```python
from build123d import *

# Parameters (mm, degrees)
F1_DEPTH  = 30
F0_W      = 37.5
F0_H      = 10
F2_DEPTH  = 100
F4_DEPTH  = 70
F5_W      = 20.9091625453
F5_H      = 25
F6_DEPTH  = 70
F7_DEPTH  = 70
F9_DEPTH  = 5
F12_DEPTH = 17.5


with BuildPart() as f1:
    # F0 (on Right) → F1 (new body)
    with BuildSketch(Plane.YZ):
        with BuildLine():
            Line((-100, 15), (-100, 0))
            Line((-100, 0), (-50, 0))
            Line((-50, 0), (-12.5, 0))
            Line((-12.5, 0), (12.5, 0))
            Line((12.5, 0), (50, 0))
            Line((50, 0), (100, 0))
            Line((100, 0), (100, 40))
            Line((100, 40), (40, 40))
            ThreePointArc((40, 40), (20.4711584909, 13.3855671691), (-12.5, 15))
            Line((-12.5, 15), (-100, 15))
        make_face()
    extrude(amount=-F1_DEPTH)

    # F0 (on Right) → F2 (join)
    with BuildSketch(Plane.YZ):
        with Locations((-31.25, -5)):
            Rectangle(F0_W, F0_H)
        with Locations((31.25, -5)):
            Rectangle(F0_W, F0_H)
    extrude(amount=-F2_DEPTH)

    # F3 (on face) → F4 (join)
    with BuildSketch(Plane(origin=(-30, 0, 0), x_dir=(0, -1, 0), z_dir=(-1, 0, 0))):
        with BuildLine():
            Line((12.5, 15), (-23.473678133, 15))
            ThreePointArc((-23.473678133, 15), (-34.5610974405, 25.633015883), (-40, 40))
            Line((-40, 40), (-100, 40))
            Line((-100, 40), (-100, 0))
            Line((-100, 0), (-50, 0))
            Line((-50, 0), (-12.5, 0))
            Line((-12.5, 0), (12.5, 0))
            Line((12.5, 0), (50, 0))
            Line((50, 0), (100, 0))
            Line((100, 0), (100, 15))
            Line((100, 15), (12.5, 15))
        make_face()
    extrude(amount=F4_DEPTH)

    # F5 (on face) → F6 (join)
    with BuildSketch(Plane(origin=(-100, 0, 0), x_dir=(0, -1, 0), z_dir=(-1, 0, 0))):
        with BuildLine():
            Line((-23.473678133, 15), (-5.478678133, 15))
            Line((-5.478678133, 15), (-38.6573392432, 34.1557089233))
            ThreePointArc((-38.6573392432, 34.1557089233), (-32.7999061901, 23.2030943833), (-23.473678133, 15))
        make_face()
        with Locations((-89.5454187273, 27.5)):
            Rectangle(F5_W, F5_H)
        Polygon((-79.0908374547, 40), (-48.7799483222, 40), (-79.0908374547, 57.5), align=None)
    extrude(amount=-F6_DEPTH)

    # F5 (on face) → F7 (cut)
    with BuildSketch(Plane(origin=(-100, 0, 0), x_dir=(0, -1, 0), z_dir=(-1, 0, 0))):
        with BuildLine():
            Line((-48.7799483222, 40), (-38.6573392432, 34.1557089233))
            ThreePointArc((-38.6573392432, 34.1557089233), (-39.4545948044, 37.048924554), (-40, 40))
            Line((-40, 40), (-48.7799483222, 40))
        make_face()
    extrude(amount=-F7_DEPTH, mode=Mode.SUBTRACT)

    # F8 (on face) → F9 (cut)
    with BuildSketch(Plane(origin=(0, -5.1255209951, 8.8776627788), x_dir=(1, 0, 0), z_dir=(0, -0.5, 0.8660254038))):
        with BuildLine():
            Line((-85.9351158142, 57.2446744423), (-76.4564392374, 57.2446744423))
            ThreePointArc((-76.4564392374, 57.2446744423), (-77.5, 62.2446744423), (-76.4564392374, 67.2446744423))
            Line((-76.4564392374, 67.2446744423), (-85.9351158142, 67.2446744423))
            Line((-85.9351158142, 67.2446744423), (-99.6410161514, 67.2446744423))
            ThreePointArc((-99.6410161514, 67.2446744423), (-99.9101386799, 64.7511096302), (-100, 62.2446744423))
            ThreePointArc((-100, 62.2446744423), (-99.9101386799, 59.7382392545), (-99.6410161514, 57.2446744423))
            Line((-99.6410161514, 57.2446744423), (-85.9351158142, 57.2446744423))
        make_face()
        with BuildLine():
            Line((-60, 73.7011136797), (-60, 96.8856905937))
            ThreePointArc((-60, 96.8856905937), (-62.4935647997, 97.1548131213), (-64.999999975, 97.2446744423))
            ThreePointArc((-64.999999975, 97.2446744423), (-67.5064351754, 97.1548131231), (-70, 96.8856905937))
            Line((-70, 96.8856905937), (-70, 73.7011136797))
            ThreePointArc((-70, 73.7011136797), (-65, 74.7446744423), (-60, 73.7011136797))
        make_face()
        with BuildLine():
            Line((-70, 12.2446744423), (-60, 12.2446744423))
            Line((-60, 12.2446744423), (-60, 50.7882352049))
            ThreePointArc((-60, 50.7882352049), (-65, 49.7446744423), (-70, 50.7882352049))
            Line((-70, 50.7882352049), (-70, 12.2446744423))
        make_face()
        with BuildLine():
            ThreePointArc((-30.3589838486, 57.2446744423), (-30.0898613201, 59.7382392545), (-30, 62.2446744423))
            ThreePointArc((-30, 62.2446744423), (-30.0898613201, 64.7511096302), (-30.3589838486, 67.2446744423))
            Line((-30.3589838486, 67.2446744423), (-53.5435607626, 67.2446744423))
            ThreePointArc((-53.5435607626, 67.2446744423), (-52.7636710884, 64.7985449884), (-52.5, 62.2446744423))
            ThreePointArc((-52.5, 62.2446744423), (-52.7636710884, 59.6908038962), (-53.5435607626, 57.2446744423))
            Line((-53.5435607626, 57.2446744423), (-30.3589838486, 57.2446744423))
        make_face()
        with BuildLine():
            ThreePointArc((-64.999999975, 97.2446744423), (-62.4935647997, 97.1548131213), (-60, 96.8856905937))
            Line((-60, 96.8856905937), (-60, 97.2446744423))
            Line((-60, 97.2446744423), (-64.999999975, 97.2446744423))
        make_face()
        with BuildLine():
            ThreePointArc((-70, 96.8856905937), (-67.5064351754, 97.1548131231), (-64.999999975, 97.2446744423))
            Line((-64.999999975, 97.2446744423), (-70, 97.2446744423))
            Line((-70, 97.2446744423), (-70, 96.8856905937))
        make_face()
        with BuildLine():
            Line((-100, 67.2446744423), (-100, 62.2446744423))
            ThreePointArc((-100, 62.2446744423), (-99.9101386799, 64.7511096302), (-99.6410161514, 67.2446744423))
            Line((-99.6410161514, 67.2446744423), (-100, 67.2446744423))
        make_face()
        with BuildLine():
            Line((-100, 62.2446744423), (-100, 57.2446744423))
            Line((-100, 57.2446744423), (-99.6410161514, 57.2446744423))
            ThreePointArc((-99.6410161514, 57.2446744423), (-99.9101386799, 59.7382392545), (-100, 62.2446744423))
        make_face()
        with BuildLine():
            ThreePointArc((-30.3589838486, 67.2446744423), (-30.0898613201, 64.7511096302), (-30, 62.2446744423))
            Line((-30, 62.2446744423), (-30, 67.2446744423))
            Line((-30, 67.2446744423), (-30.3589838486, 67.2446744423))
        make_face()
        with BuildLine():
            Line((-30.3589838486, 57.2446744423), (-30, 57.2446744423))
            Line((-30, 57.2446744423), (-30, 62.2446744423))
            ThreePointArc((-30, 62.2446744423), (-30.0898613201, 59.7382392545), (-30.3589838486, 57.2446744423))
        make_face()
        with BuildLine():
            ThreePointArc((-70, 50.7882352049), (-65, 49.7446744423), (-60, 50.7882352049))
            ThreePointArc((-60, 50.7882352049), (-56.1611652352, 53.4058396775), (-53.5435607626, 57.2446744423))
            ThreePointArc((-53.5435607626, 57.2446744423), (-52.7636710884, 59.6908038962), (-52.5, 62.2446744423))
            ThreePointArc((-52.5, 62.2446744423), (-52.7636710884, 64.7985449884), (-53.5435607626, 67.2446744423))
            ThreePointArc((-53.5435607626, 67.2446744423), (-56.1611652352, 71.0835092071), (-60, 73.7011136797))
            ThreePointArc((-60, 73.7011136797), (-65, 74.7446744423), (-70, 73.7011136797))
            ThreePointArc((-70, 73.7011136797), (-73.8388347648, 71.0835092071), (-76.4564392374, 67.2446744423))
            ThreePointArc((-76.4564392374, 67.2446744423), (-77.5, 62.2446744423), (-76.4564392374, 57.2446744423))
            ThreePointArc((-76.4564392374, 57.2446744423), (-73.8388347648, 53.4058396775), (-70, 50.7882352049))
        make_face()
    extrude(amount=-F9_DEPTH, mode=Mode.SUBTRACT)

    # F11 (on offset) → F12 (cut)
    with BuildSketch(Plane.XY.offset(57.5)):
        with BuildLine():
            add(Edge.make_bspline(
                [(-65, 79.0908374547), (-100, 79.0908374547), (-100, 48.7799483222)],
                knots=[4.7123889804, 4.7123889804, 4.7123889804, 6.2831853072, 6.2831853072, 6.2831853072], degree=2, weights=[1, 0.7071067812, 1]))
            Line((-65, 79.0908374547), (-100, 79.0908374547))
            Line((-100, 79.0908374547), (-100, 48.7799483222))
        make_face()
        with BuildLine():
            Line((-30, 48.7799483222), (-30, 79.0908374547))
            Line((-30, 79.0908374547), (-65, 79.0908374547))
            add(Edge.make_bspline(
                [(-30, 48.7799483222), (-30, 79.0908374547), (-65, 79.0908374547)],
                knots=[3.1415926536, 3.1415926536, 3.1415926536, 4.7123889804, 4.7123889804, 4.7123889804], degree=2, weights=[1, 0.7071067812, 1]))
        make_face()
    extrude(amount=-F12_DEPTH, mode=Mode.SUBTRACT)


solid = f1.part
```
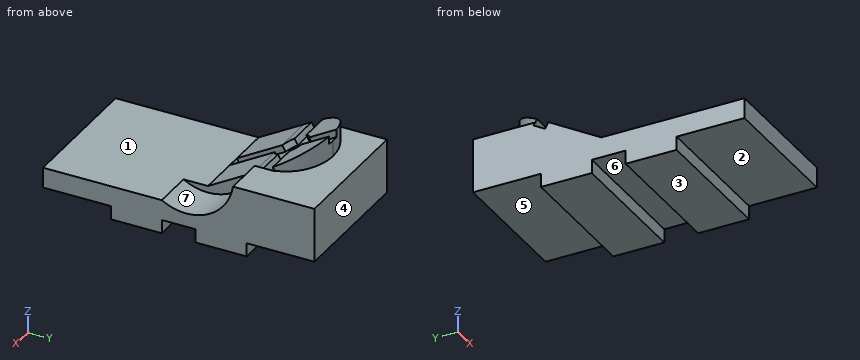
Geometry: final body of the model. Coordinates: model frame, mm. Face numbers are marked on the shaded views. A direction names the side the tool comes from. Coordinates: 2 decimals unless noted, no trailing zeros. Order: outer loops, then holes, each group sorted by start corner. A loop starts at its lowest first (then second) coordinate and runs counter-clockwise, first axis right, second up.
Item 1: Contact query for flat-ended pins moving along their axis: P1, Ø1.5, axis at x = -36.5, y = 21.5, coming from the +Z side; P2, Ø7, axis at y = 15.5, z = 18.5, coming from the +X side; P3, Ø12, axis at x = -12.5, y = -28, coming from the +Z side. Output: stop coordinate, or through.
Answer:
P1: stops at z = 24.68
P2: stops at x = -30
P3: stops at z = 15
Item 2: Section query A-A (x = -7). Output: boundary loops of the cut face in (y, z), then the cut area to 3 significant figures.
Answer:
outline: (-100, 0) - (-50, 0) - (-50, -10) - (-12.5, -10) - (-12.5, 0) - (12.5, 0) - (12.5, -10) - (50, -10) - (50, 0) - (100, 0) - (100, 40) - (40, 40) arc R34.85 cw to (-12.5, 15) - (-100, 15) - close
area: 5,270 mm2
Item 3: Access query for the marked faces 1, 2 and 3. Directions: +Z, -Z, +X, -X, +Y, -Y. A direction counts if a zero-diameter tool reaches every point of the face in a straight line with its end or side. Return the directions, or none.
Answer:
face 1: +Z, +X, -X, -Y
face 2: -Z, +X, -X, -Y
face 3: -Z, +X, -X, +Y, -Y
Item 4: Section query C-C (y = -66). Output: boundary loops of the cut face in (x, z).
Answer:
outline: (-100, 0) - (0, 0) - (0, 15) - (-100, 15) - close
Item 5: Section query B-B (z = 23.5). Output: boundary loops of the cut face in (x, y), then the cut area to 3 significant figures.
Answer:
outline: (-100, 20.2) - (-70, 20.2) - (-70, 30.2) - (-60, 30.2) - (-60, 20.2) - (-30, 20.2) - (-30, 33.03) - (0, 33.03) - (0, 100) - (-100, 100) - close
area: 7,490 mm2
Item 6: Section query D-D (y = -21). Output: boundary loops of the cut face in (x, z).
Answer:
outline: (-100, -10) - (0, -10) - (0, 15) - (-100, 15) - close
Item 7: Draft query along Y for the marked faces 4, 5, 6 and 7. Return one class per face: released by +Y, released by -Y, zero draft, split by the parting line, or undercut.
Answer:
face 4: released by +Y
face 5: zero draft
face 6: undercut
face 7: undercut
Item 8: Material intervals for line 1 along Z through (x, y) = (-87, -65.5); line 2 along Y through (x, z) = (-75, -2); line 3 along Z through (x, y) = (-81.5, -24), sorted ascending.
Answer:
line 1: z = 0 to 15
line 2: y = -50 to -12.5, 12.5 to 50
line 3: z = -10 to 15
